The drawing under review shows one solid part. Ordinate dimensions are in mm from its lowest x, y, z. A direction names the side the tool comes from. Round coordinates to 2 decimals unless told otherwise and drop trailing zeros. Write each loop counter-clockwise with the first axis right and the second up, starting at its lowest first coordinate (ties: lowest second). Pieces come first, ordered by that corner, then holes. Notation, with made-up numbers: M 20,58 L 40,58 A11 ccw 40,74 Z; hole C -31.5,26.5 d11. An arc over 180 degrees is marked long. Write item = value, one per line. Start each with the question number.
Item 1: Tool access review of the marked faces 1 and 2: name each direction out of +Z, -Z, +X, -X, +Y, -Y from which nothing blocks a thin tool from reaching the whole face with its end or side.
Item 2: Take a section at C-C, the plane z = 3.85. Give the boundary of the cut face in (x, y).
Item 3: Take a section at A-A, the plane y = 4.5. Give the boundary of the cut face in (x, z).
Item 4: To check wall thickness, follow line 1 along X through (y, z) = (5.5, 1.9); line 2 along Y through (x, z) = (25, 2.2); line 3 along X through (y, z) = (16.75, 3.15) (1 decimal). State the ranges of each line that lie inside material, in increasing order.
Item 5: Take a section at D-D, the plane y = 1.25. Give the boundary of the cut face in (x, z).
Item 6: Take a section at B-B, the plane x = 31.5. Give the boundary of the cut face in (y, z), plus the area to 3 significant figures.
Item 7: The part is to be moulded in two halves that separate along X. For the marked faces 3, 4, 5 and 6, say which applies: +X half, -X half, draft (parallel to the pull), parting line (faces both ways), or undercut.
Item 8: For pin 1 Ø1.8 at (x, y) = (2.91, 17.14) entering from -Z, flat-tipped, find the tip position at first contact; note if it passes through.
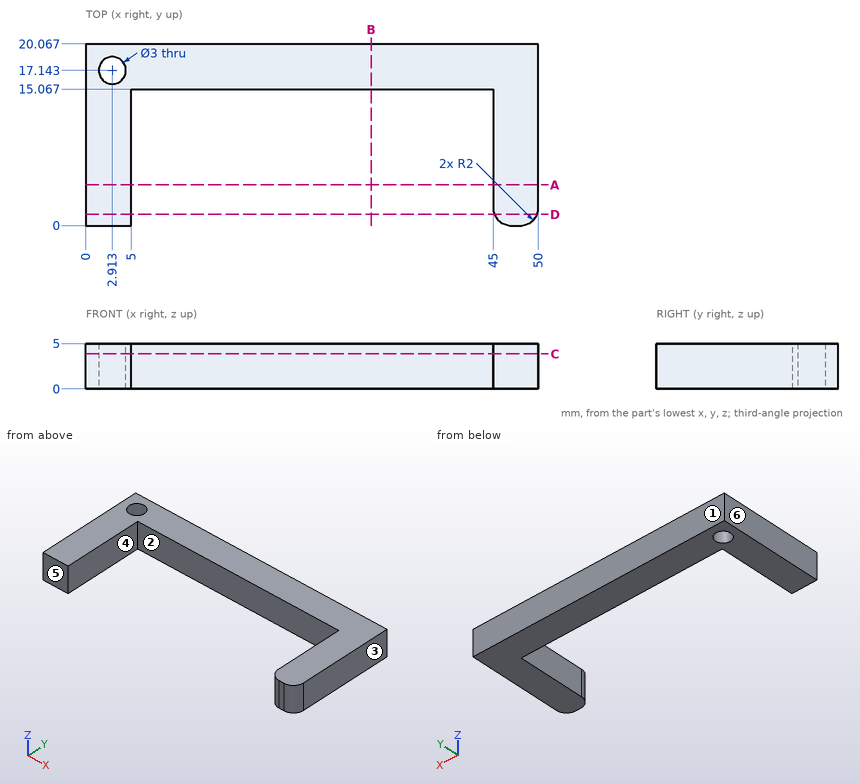
Response values:
q1.face_1 = +Z, -Z, +X, -X, +Y
q1.face_2 = +Z, -Z, -Y
q2.outline = M 0,0 L 5,0 L 5,15.07 L 45,15.07 L 45,2 A2 ccw 47,0 L 48,0 A2 ccw 50,2 L 50,20.07 L 0,20.07 Z; hole C 2.91,17.14 d3
q3.outline = M 0,0 L 5,0 L 5,5 L 0,5 Z; M 45,0 L 50,0 L 50,5 L 45,5 Z
q4.line_1 = 0 to 5, 45 to 50
q4.line_2 = 15.07 to 20.07
q4.line_3 = 0 to 1.5, 4.4 to 50
q5.outline = M 0,0 L 5,0 L 5,5 L 0,5 Z; M 45.15,0 L 49.85,0 L 49.85,5 L 45.15,5 Z
q6.outline = M 15.07,0 L 20.07,0 L 20.07,5 L 15.07,5 Z
q6.area = 25.0 mm2
q7.face_3 = +X half
q7.face_4 = undercut
q7.face_5 = draft
q7.face_6 = -X half
q8.pin_1 = through
